```python
from build123d import *

# Parameters (mm, degrees)
BOSS_EXTRUDE2_DEPTH = 5
BOSS_EXTRUDE3_START = 25
BOSS_EXTRUDE3_DEPTH = 25
SKETCH7_R           = 2.55
CUT_EXTRUDE1_DEPTH  = 313.685484953


with BuildPart() as part:
    # Sketch4 → Boss-Extrude2 (new body)
    with BuildSketch(Plane.XY.offset(304.8)):
        with BuildLine():
            Line((35.5, 1.5), (35.5, 14.65))
            ThreePointArc((35.5, 14.65), (34.035533906, 18.185533906), (30.5, 19.65))
            Line((30.5, 19.65), (1.5, 19.65))
            ThreePointArc((1.5, 19.65), (-2.035533906, 18.185533906), (-3.5, 14.65))
            Line((-3.5, 14.65), (-3.5, 1.5))
            ThreePointArc((-3.5, 1.5), (-2.035533906, -2.035533906), (1.5, -3.5))
            Line((1.5, -3.5), (30.5, -3.5))
            ThreePointArc((30.5, -3.5), (34.035533906, -2.035533906), (35.5, 1.5))
        make_face()
    extrude(amount=BOSS_EXTRUDE2_DEPTH)

    # Sketch6 → Boss-Extrude3 (add)
    with BuildSketch(Plane(origin=(0, 0, 304.8), x_dir=(-1, 0, 0), z_dir=(0, 0, -1)).offset(BOSS_EXTRUDE3_START)):
        with BuildLine():
            Line((-30.5, -3.5), (-1.5, -3.5))
            ThreePointArc((-1.5, -3.5), (2.035533906, -2.035533906), (3.5, 1.5))
            Line((3.5, 1.5), (3.5, 14.65))
            ThreePointArc((3.5, 14.65), (2.035533906, 18.185533906), (-1.5, 19.65))
            Line((-1.5, 19.65), (-30.5, 19.65))
            ThreePointArc((-30.5, 19.65), (-34.035533906, 18.185533906), (-35.5, 14.65))
            Line((-35.5, 14.65), (-35.5, 1.5))
            ThreePointArc((-35.5, 1.5), (-34.035533906, -2.035533906), (-30.5, -3.5))
        make_face()
        with BuildLine():
            Line((-1.5, 17.85), (-30.5, 17.85))
            ThreePointArc((-30.5, 17.85), (-32.7627417, 16.9127417), (-33.7, 14.65))
            Line((-33.7, 14.65), (-33.7, 1.5))
            ThreePointArc((-33.7, 1.5), (-32.7627417, -0.7627417), (-30.5, -1.7))
            Line((-30.5, -1.7), (-1.5, -1.7))
            ThreePointArc((-1.5, -1.7), (0.7627417, -0.7627417), (1.7, 1.5))
            Line((1.7, 1.5), (1.7, 14.65))
            ThreePointArc((1.7, 14.65), (0.7627417, 16.9127417), (-1.5, 17.85))
        make_face(mode=Mode.SUBTRACT)
    extrude(amount=-BOSS_EXTRUDE3_DEPTH)

    # Sketch7 → Cut-Extrude1 (cut, through all)
    with BuildSketch(Plane(origin=(0, 19.65, 0), x_dir=(1, 0, 0), z_dir=(0, 1, 0))):
        with Locations(Location((16, -296.8, 0), (0, 0, 180))):
            Circle(SKETCH7_R)
        with Locations(Location((26, -284.8, 0), (0, 0, 180))):
            Circle(SKETCH7_R)
        with Locations(Location((6, -284.8, 0), (0, 0, 180))):
            Circle(SKETCH7_R)
    extrude(amount=-CUT_EXTRUDE1_DEPTH, mode=Mode.SUBTRACT)


solid = part.part
```
Build history of the part. All positions in model axes, mm. A direction names the side the tool comes from. Round coordinates to 2 decimals unless told otherwise and drop trailing zeros. Loops run counter-clockwise (first coordinate to the right, second up) from the corner with the lowest first, then second, coordinate; pieces in that order, holes last.
Item 1: Which spindle directions (+Z, -Z, +X, -X, +Y, -Y) get a long thin tool onto all of the face, cutting with end or side? Do faces 1 (the face through (-2.07, 18.15, 294.59)), 2 (the face through (16, 17.85, 292)). Say none if no direction does.
Item 2: Saw through at A-A (z = 284.8). State how many separate pieces and enclosed holes the cut face has, then the cut area to 3 significant figures.
Item 3: Saw through at B-B (z = 296.8). List the corners of the cut face in (x, y), then the cut area to 3 significant figures.
Item 4: Two-plate mould, pull along Y, no slides. Class faces 3 (the face through (34.07, -2, 294.59)), 4 (the face through (19, 19.65, 295)), 5 (the face through (35.5, 8, 295)), 6 (the face through (-0.738, -0.787, 292.125)): released by +Y, released by -Y, zero draft, split by the parting line, or undercut.
Item 5: Saw through at D-D (y = 4.25). List the corners of the cut face in (x, z).
Item 6: Drill centre lines: line 1 along Y through (x, z) = (25.5, 292.75); line 2 along Z through (x, y) = (26, 19.1); line 3 along X through (y, z) = (10, 283.5). Where is each one in solid material? Low to high.
Item 7: Pin check, flat tips, straight feed: P1, Ø4, axis at y = 17, z = 285.5, coming from the +X side; P2, Ø12, axis at x = 11, y = 6.5, coming from the -Z side; P3, Ø4.5, axis at x = 6, z = 284.8, coming from the +Y side. Stop position of each tip, or through.
Item 8: Saw through at C-C (x = 24). List the corners of the cut face in (y, z), then the cut area to 3 significant figures.
Worked answers:
1. face 1: +Z, -Z, -X, +Y
1. face 2: -Z
2. separate pieces: 4
2. enclosed holes: 0
2. area: 161 mm2
3. outline: (-3.5, 1.5) arc R5 ccw to (1.5, -3.5) - (13.45, -3.5) - (13.45, -1.7) - (1.5, -1.7) arc R3.2 cw to (-1.7, 1.5) - (-1.7, 14.65) arc R3.2 cw to (1.5, 17.85) - (13.45, 17.85) - (13.45, 19.65) - (1.5, 19.65) arc R5 ccw to (-3.5, 14.65) - close; (18.55, -3.5) - (30.5, -3.5) arc R5 ccw to (35.5, 1.5) - (35.5, 14.65) arc R5 ccw to (30.5, 19.65) - (18.55, 19.65) - (18.55, 17.85) - (30.5, 17.85) arc R3.2 cw to (33.7, 14.65) - (33.7, 1.5) arc R3.2 cw to (30.5, -1.7) - (18.55, -1.7) - close
3. area: 180 mm2
4. face 3: released by -Y
4. face 4: released by +Y
4. face 5: zero draft
4. face 6: undercut
5. outline: (-3.5, 279.8) - (-1.7, 279.8) - (-1.7, 304.8) - (33.7, 304.8) - (33.7, 279.8) - (35.5, 279.8) - (35.5, 309.8) - (-3.5, 309.8) - close
6. line 1: y = -3.5 to -1.7, 17.85 to 19.65
6. line 2: z = 279.8 to 282.25, 287.35 to 309.8
6. line 3: x = -3.5 to -1.7, 33.7 to 35.5
7. P1: stops at x = 35.49
7. P2: stops at z = 304.8
7. P3: passes through
8. outline: (-3.5, 279.8) - (-1.7, 279.8) - (-1.7, 283.22) - (-3.5, 283.22) - close; (-3.5, 286.38) - (-1.7, 286.38) - (-1.7, 304.8) - (17.85, 304.8) - (17.85, 286.38) - (19.65, 286.38) - (19.65, 309.8) - (-3.5, 309.8) - close; (17.85, 279.8) - (19.65, 279.8) - (19.65, 283.22) - (17.85, 283.22) - close
8. area: 194 mm2
